Verification items for the finished model (mm, model axes). A direction names the side the tool comes from. Give positions to 0.01 mm unless a question says otherwise; leave off trailing zeros. Write each loop counter-clockwise with the first axis right and the second up, starting at its lowest first coordinate (ties: lowest second). Pieces come first, ordered by that corner, then holes. Notation, with made-up numbers: M 32.25,68 L 69.25,68 A19 ccw 69.25,78 Z; hole C 89.5,88 d11. An arc over 180 degrees is marked long. Write item = value, one per line.
from build123d import *

# Parameters (mm, degrees)
PAD_DEPTH    = 4
SKETCH001_R  = 1.25
POCKET_DEPTH = 9.001


with BuildPart() as part:
    # Sketch → Pad (new body)
    with BuildSketch(Plane.XY):
        with BuildLine():
            Line((0, 0), (4, 0))
            Line((4, 0), (4, 4.5))
            ThreePointArc((5.5, 6), (4.43934, 5.56066), (4, 4.5))
            Line((5.5, 6), (10.5, 6))
            ThreePointArc((12, 4.5), (11.56066, 5.56066), (10.5, 6))
            Line((12, 4.5), (12, 0))
            Line((12, 0), (15, 0))
            Line((15, 0), (15, 4.5))
            ThreePointArc((15, 4.5), (13.681981, 7.681981), (10.5, 9))
            Line((0, 9), (10.5, 9))
            Line((0, 9), (0, 0))
        make_face()
    extrude(amount=PAD_DEPTH)

    # Sketch001 (on Face2 of Pad) → Pocket (cut, through all)
    with BuildSketch(Plane.XZ):
        with Locations((2, 2)):
            Circle(SKETCH001_R)
    extrude(amount=-POCKET_DEPTH, mode=Mode.SUBTRACT)


solid = part.part
1) Cross-section at D-D on z = 3.45. Record the boundary of the cut face in (x, y), plus the area to 3 significant figures.
From the geometry:
outline = M 0,0 L 4,0 L 4,4.5 A1.5 cw 5.5,6 L 10.5,6 A1.5 cw 12,4.5 L 12,0 L 15,0 L 15,4.5 A4.5 ccw 10.5,9 L 0,9 Z
area = 83.6 mm^2
2) Depth check by flat-ended pin: P1, Ø1.2, axis at y = 2, z = 2.5, coming from the -X side; P2, Ø2, axis at x = 10, y = 4, coming from the -Z side; P3, Ø1.5, axis at y = 6, z = 3, coming from the +X side; P4, Ø2, axis at x = 7.5, z = 1.5, coming from the -Y side. Enter the tip coordinate at first touch or a pass-through.
From the geometry:
P1 = 0
P2 = through
P3 = 14.94
P4 = 6
3) Cross-section at A-A on y = 3.75. Record the boundary of the cut face in (x, z).
From the geometry:
outline = M 0,0 L 4,0 L 4,4 L 0,4 Z; M 12,0 L 15,0 L 15,4 L 12,4 Z; hole C 2,2 d2.5
4) Draft check along Z on faces 1 (the flat face through (1, 0, 1)), 2 (the flat face through (7, 7, 4)), 3 (the cylindrical face through (3.19, 4.44, 2.38)). Enter one of: +Z half, -Z half, draft (parallel to the pull), parting line (faces both ways), or undercut.
From the geometry:
face_1 = draft
face_2 = +Z half
face_3 = undercut
5) Cross-section at C-C on z = 2. Record the boundary of the cut face in (x, y).
From the geometry:
outline = M 0,0 L 0.75,0 L 0.75,9 L 0,9 Z; M 3.25,0 L 4,0 L 4,4.5 A1.5 cw 5.5,6 L 10.5,6 A1.5 cw 12,4.5 L 12,0 L 15,0 L 15,4.5 A4.5 ccw 10.5,9 L 3.25,9 Z
6) Cross-section at B-B on x = 2. Record the boundary of the cut face in (y, z).
From the geometry:
outline = M 0,0 L 9,0 L 9,0.75 L 0,0.75 Z; M 0,3.25 L 9,3.25 L 9,4 L 0,4 Z
7) Tool access check on faces 4 (the cylindrical face through (4.45, 5.57, 1.97)), 5 (the flat face through (13, 0, 2)). Record the directions out of +Z, -Z, +X, -X, +Y, -Y that give a thin tool (end or side, any length) a straight path to the whole face; none if there is none.
From the geometry:
face_4 = +Z, -Z, -Y
face_5 = +Z, -Z, +X, -X, -Y
8) Material ranges on probe 1 along X at (y, z) = (3, 0.25); probe 2 along Z at (x, y) = (2, 7); probe 3 along X at (y, z) = (4.5, 1.3), recorded low to high. Write a range as from..to.
From the geometry:
probe_1 = 0..4, 12..15
probe_2 = 0..0.75, 3.25..4
probe_3 = 0..0.96, 3.04..4, 12..15
